Check sheet for the modelled part. Datum: model origin and axes. Units: mm. Face numbers are marked on the shaded views. A direction names the side the tool comes from. Round coordinates to 2 decimals unless told otherwise and drop trailing zeros. Write each loop counter-clockwise with the first axis right and the second up, starting at its lowest first coordinate (ties: lowest second). Pieces come first, ordered by that corner, then holes. Notation, with made-up numbers: M -33.75,-20.5 L -17.75,-20.5 A8 ccw -17.75,-8.5 Z; hole C 74.25,64 d2. An arc over 180 degrees is marked long. Put each result on its own line as item: value.
```python
from build123d import *

# Parameters (mm, degrees)
SKETCH1_W           = 130
SKETCH1_H           = 97
BOSS_EXTRUDE1_DEPTH = 70
SKETCH2_W           = 78
SKETCH2_H           = 50
CUT_EXTRUDE1_DEPTH  = 137.1396342
FILLET3_R           = 5
SKETCH3_R           = 5.2
CUT_EXTRUDE2_DEPTH  = 108.131928014
SKETCH4_R           = 6.5
CUT_EXTRUDE3_DEPTH  = 5
FILLET2_R           = 5
FILLET4_R           = 2


with BuildPart() as part:
    # Sketch1 → Boss-Extrude1 (new body)
    with BuildSketch(Plane(origin=(0, 0, 0), x_dir=(1, 0, 0), z_dir=(0, 1, 0))):
        Rectangle(SKETCH1_W, SKETCH1_H)
    extrude(amount=BOSS_EXTRUDE1_DEPTH)

    # Sketch2 → Cut-Extrude1 (cut, through all)
    with BuildSketch(Plane.XY.offset(48.5)):
        with Locations((0, 25)):
            Rectangle(SKETCH2_W, SKETCH2_H)
    extrude(amount=-CUT_EXTRUDE1_DEPTH, mode=Mode.SUBTRACT)

    # Fillet3
    fillet3_edges = [part.edges().sort_by_distance(p)[0] for p in [
        (-39, 50, 0),
        (39, 50, 0),
    ]]
    fillet(fillet3_edges, radius=FILLET3_R)

    # Sketch3 → Cut-Extrude2 (cut, through all)
    with BuildSketch(Plane(origin=(0, 70, 0), x_dir=(1, 0, 0), z_dir=(0, 1, 0))):
        with Locations(Location((0, 0, 0), (0, 0, 270))):
            Circle(SKETCH3_R)
    extrude(amount=-CUT_EXTRUDE2_DEPTH, mode=Mode.SUBTRACT)

    # Sketch4 → Cut-Extrude3 (cut)
    with BuildSketch(Plane(origin=(0, 70, 0), x_dir=(1, 0, 0), z_dir=(0, 1, 0))):
        with Locations(Location((0, 0, 0), (0, 0, 270))):
            Circle(SKETCH4_R)
    extrude(amount=-CUT_EXTRUDE3_DEPTH, mode=Mode.SUBTRACT)

    # Fillet2
    fillet2_edges = [part.edges().sort_by_distance(p)[0] for p in [
        (-65, 35, 48.5),
        (-65, 35, -48.5),
        (65, 35, -48.5),
        (65, 35, 48.5),
    ]]
    fillet(fillet2_edges, radius=FILLET2_R)

    # Fillet4
    fillet4_edges = [part.edges().sort_by_distance(p)[0] for p in [
        (-39, 0, 0),
        (39, 0, 0),
    ]]
    fillet(fillet4_edges, radius=FILLET4_R)


solid = part.part
```
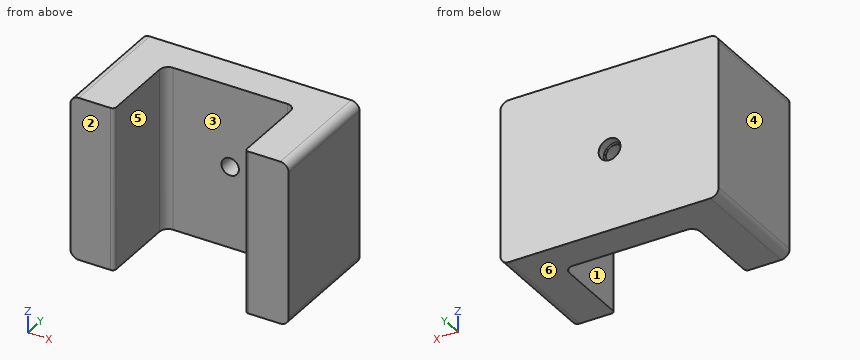
1. Depth check by flat-ended pin: pin 1 Ø8.5 at (x, z) = (0, 0) entering from +Y; pin 2 Ø5 at (x, z) = (-31.5, 9.5) entering from -Y; pin 3 Ø3 at (x, z) = (37, -6.5) entering from -Y. Enter the tip coordinate at first touch or a pass-through.
Computed values:
pin 1: passes through
pin 2: stops at y = 50
pin 3: stops at y = 47.18
2. Cross-section at A-A (z = 0). Enter the section's corners in (x, y), then the cut area to 3 significant figures.
Computed values:
outline: M -65,0 L -41,0 A2 ccw -39,2 L -39,45 A5 cw -34,50 L -5.2,50 L -5.2,65 L -6.5,65 L -6.5,70 L -65,70 Z; M 5.2,50 L 34,50 A5 cw 39,45 L 39,2 A2 ccw 41,0 L 65,0 L 65,70 L 6.5,70 L 6.5,65 L 5.2,65 Z
area: 4,990 mm2
3. Access from +Z, -Z, +X, -X, +Y, -Y to the whole of each face (thin tool, end or side, straight path). Record for the marked faces 5 and 6.
Computed values:
face 5: +Z, -Z, -Y
face 6: -Z, +X, -X, +Y, -Y
4. Cross-section at D-D (z = -29.5). Enter the section's corners in (x, y), then the cut area to 3 significant figures.
Computed values:
outline: M -65,0 L -41,0 A2 ccw -39,2 L -39,45 A5 cw -34,50 L 34,50 A5 cw 39,45 L 39,2 A2 ccw 41,0 L 65,0 L 65,70 L -65,70 Z
area: 5,210 mm2
5. Cross-section at B-B (y = 10). Enter the section's corners in (x, z).
Computed values:
outline: M -65,-43.5 A5 ccw -60,-48.5 L -39,-48.5 L -39,48.5 L -60,48.5 A5 ccw -65,43.5 Z; M 39,-48.5 L 60,-48.5 A5 ccw 65,-43.5 L 65,43.5 A5 ccw 60,48.5 L 39,48.5 Z
6. Scan lines: probe 1 along X at (y, z) = (66.3, 0); probe 2 along X at (y, z) = (37, 37); probe 3 along Y at (x, z) = (-31.5, -21). Record each from-to range of solid material in increasing order.
Computed values:
probe 1: x = -65 to -6.5, 6.5 to 65
probe 2: x = -65 to -39, 39 to 65
probe 3: y = 50 to 70
7. Cross-section at C-C (x = 0). Enter the section's corners in (y, z).
Computed values:
outline: M 50,-48.5 L 70,-48.5 L 70,-6.5 L 65,-6.5 L 65,-5.2 L 50,-5.2 Z; M 50,5.2 L 65,5.2 L 65,6.5 L 70,6.5 L 70,48.5 L 50,48.5 Z
8. Release check for a two-part mould opening along X. For the marked faces 1, 2, 3 and 4 record: +X half, -X half, draft (parallel to the pull), parting line (faces both ways), or undercut.
Computed values:
face 1: undercut
face 2: draft
face 3: undercut
face 4: -X half
